```python
from build123d import *

# Parameters (mm, degrees)
F0_W      = 69.85
F0_H      = 12.7
F1_DEPTH  = 25.4
F3_DEPTH  = 12.7
F5_DEPTH  = 25.4
F6_DEPTH  = 12.7
F7_R      = 6.35
F8_DEPTH  = 38.1
F10_DEPTH = 12.7


with BuildPart() as f1:
    # F0 (on Front) → F1 (new body)
    with BuildSketch(Plane.XZ):
        with Locations((34.925, 6.35)):
            Rectangle(F0_W, F0_H)
    extrude(amount=F1_DEPTH)

    # F2 (on face) → F3 (cut)
    with BuildSketch(Plane.XY.offset(12.7)):
        with BuildLine():
            ThreePointArc((38.1, -12.7), (36.2401280605, -8.2098719395), (31.75, -6.35))
            ThreePointArc((31.75, -6.35), (25.4, -12.7), (31.75, -19.05))
            ThreePointArc((31.75, -19.05), (36.2401280605, -17.1901280605), (38.1, -12.7))
        make_face()
        with BuildLine():
            ThreePointArc((57.15, -19.05), (50.8, -12.7), (57.15, -6.35))
            Line((57.15, -6.35), (31.75, -6.35))
            ThreePointArc((31.75, -6.35), (36.2401280605, -8.2098719395), (38.1, -12.7))
            ThreePointArc((38.1, -12.7), (36.2401280605, -17.1901280605), (31.75, -19.05))
            Line((31.75, -19.05), (57.15, -19.05))
        make_face()
        with BuildLine():
            ThreePointArc((57.15, -19.05), (61.6401280605, -17.1901280605), (63.5, -12.7))
            ThreePointArc((63.5, -12.7), (61.6401280605, -8.2098719395), (57.15, -6.35))
            ThreePointArc((57.15, -6.35), (50.8, -12.7), (57.15, -19.05))
        make_face()
    extrude(amount=-F3_DEPTH, mode=Mode.SUBTRACT)

    # F4 (on face) → F5 (join)
    with BuildSketch(Plane.XY.offset(12.7)):
        with BuildLine():
            ThreePointArc((12.7, -25.4), (21.6802561211, -21.6802561211), (25.4, -12.7))
            ThreePointArc((25.4, -12.7), (21.6802561211, -3.7197438789), (12.7, 0))
            ThreePointArc((12.7, 0), (3.7197438789, -3.7197438789), (0, -12.7))
            ThreePointArc((0, -12.7), (3.7197438789, -21.6802561211), (12.7, -25.4))
        make_face()
    extrude(amount=F5_DEPTH)

    # F6 (cut): faces of the model
    f6_faces = [f1.faces().sort_by_distance(p)[0] for p in [
        (2.8367728246, -2.8367728246, 12.7),
        (2.8367728246, -22.5632271754, 12.7),
    ]]
    extrude(f6_faces, amount=-F6_DEPTH, mode=Mode.SUBTRACT)

    # F7 (on face) → F8 (cut)
    with BuildSketch(Plane.XY.offset(38.1)):
        with Locations((12.7, -12.7)):
            Circle(F7_R)
    extrude(amount=-F8_DEPTH, mode=Mode.SUBTRACT)

    # F9 (on face) → F10 (cut)
    with BuildSketch(Plane.XY.offset(12.7)):
        with BuildLine():
            ThreePointArc((57.15, 0), (66.1302561211, -3.7197438789), (69.85, -12.7))
            Line((69.85, -12.7), (69.85, 0))
            Line((69.85, 0), (57.15, 0))
        make_face()
        with BuildLine():
            ThreePointArc((69.85, -12.7), (66.1302561211, -21.6802561211), (57.15, -25.4))
            Line((57.15, -25.4), (69.85, -25.4))
            Line((69.85, -25.4), (69.85, -12.7))
        make_face()
    extrude(amount=-F10_DEPTH, mode=Mode.SUBTRACT)


solid = f1.part
```
Design review of the part built by this model. Coordinates are the model's own, in mm. A direction names the side the tool comes from. Round coordinates to 2 decimals unless told otherwise and drop trailing zeros. Order: outer loops, then holes, each group sorted by start corner. A loop starts at its lowest first (then second) coordinate and runs counter-clockwise, first axis right, second up. Notation, with made-up numbers: M -27.75,41.5 L -6.75,41.5 A24 ccw -6.75,60.5 Z; hole C 32,-22.75 d10. An arc over 180 degrees is marked long. Put each result on its own line as item: value.
Q1. Consider section D-D (y = -5.5). State the section outline as (x, z) points.
Reported:
outline: M 2.24,0 L 67.61,0 L 67.61,12.7 L 23.16,12.7 L 23.16,38.1 L 2.24,38.1 Z
Q2. Insertion check: pin 1 Ø7.5 at (x, y) = (46.5, -16) entering from +Z; pin 2 Ø1.5 at (y, z) = (-20.5, 30) entering from +X; pin 3 Ø6 at (y, z) = (-21.5, 30) entering from -X. Each pin has a flat end and moves straight along its axis. Give the tip position at first contact, or say it passes through.
Reported:
pin 1: z = 12.7
pin 2: x = 23.26
pin 3: x = 1.4
Q3. Consider section A-A (x = 38.5). State the section outline as (y, z) points, and give its area (3 significant figures).
Reported:
outline: M -25.4,0 L -19.05,0 L -19.05,12.7 L -25.4,12.7 Z; M -6.35,0 L 0,0 L 0,12.7 L -6.35,12.7 Z
area: 161 mm²
Q4. Machinability: for faces 1 (the face through (35, 0, 6)), 2 (the face through (25.4, -12.6, 6.4)), which of the approach directions +Z, -Z, +X, -X, +Y, -Y give a long, thin tool a straight path to every point of the face, cutting with its end or side? Answer none if there is none.
Reported:
face 1: +Z, -Z, +X, -X, +Y
face 2: +Z, -Z
Q5. Draft analysis for pull direction Y (two halves, no side actions). For faces 3 (the face through (35, -25.4, 6)), 4 (the face through (47, -4, 12.7)), 5 (the face through (45, -6.35, 6)), state which applies: released by +Y, released by -Y, zero draft, split by the parting line, or undercut.
Reported:
face 3: released by -Y
face 4: zero draft
face 5: undercut
Q6. To check wall thickness, follow line 1 (X direction, y = -13, z = 6.5); line 2 (Y direction, x = 12.7, z = 15.5); line 3 (Z direction, x = 47, y = -23.5). State the ranges of each line that lie inside material, in increasing order.
Reported:
line 1: 0 to 6.36, 19.04 to 25.41, 63.49 to 69.85
line 2: -25.4 to -19.05, -6.35 to 0
line 3: 0 to 12.7
Q7. Consider section C-C (x = 23.5). State the section outline as (y, z) points, and give its area (3 significant figures).
Reported:
outline: M -25.4,0 L 0,0 L 0,12.7 L -6.02,12.7 L -6.02,38.1 L -19.38,38.1 L -19.38,12.7 L -25.4,12.7 Z
area: 662 mm²
Q8. Consider section B-B (z = 20.5). State the section outline as (x, y) points, and give its area (3 significant figures).
Reported:
outline: C 12.7,-12.7 d25.4; hole C 12.7,-12.7 d12.7
area: 380 mm²
